Model file for the job. Use its own axes, mm. Coordinates: 2 decimals unless noted, no trailing zeros. Write each loop counter-clockwise with the first axis right and the second up, starting at its lowest first coordinate (ties: lowest second). Pieces come first, ordered by that corner, then holes. Notation, with made-up numbers: (-11.5, 0.5) -> (44.5, 0.5) arc R21 cw to (44.5, 11.5) -> close; hole circle Ø4 at (80.25, -9). An arc over 180 degrees is marked (long way). Answer as a JSON object with one key per item and string values. Group by question number.
from build123d import *

# Parameters (mm, degrees)
SKETCH1_W           = 74.6
SKETCH1_H           = 62
BOSS_EXTRUDE1_DEPTH = 3.2
CUT_EXTRUDE1_REACH  = 5.2
SKETCH2_R           = 21.05
CUT_EXTRUDE2_REACH  = 5.2
SKETCH3_R           = 2.625


with BuildPart() as part:
    # Sketch1 → Boss-Extrude1 (new body)
    with BuildSketch(Plane(origin=(0, 0, 0), x_dir=(0, 0, -1), z_dir=(1, 0, 0))):
        with Locations((37.3, 31)):
            Rectangle(SKETCH1_W, SKETCH1_H)
    extrude(amount=BOSS_EXTRUDE1_DEPTH)

    # Sketch2 → Cut-Extrude1 (cut, up to next)
    with BuildSketch(Plane(origin=(3.2, 0, 0), x_dir=(0, 0, -1), z_dir=(1, 0, 0)), mode=Mode.PRIVATE) as cut_extrude1_sk1:
        with Locations((37.3, 31)):
            Circle(SKETCH2_R)
    cut_extrude1_tool1 = extrude(cut_extrude1_sk1.sketch, amount=-CUT_EXTRUDE1_REACH, mode=Mode.PRIVATE) & part.part
    add(cut_extrude1_tool1.solids().sort_by_distance((3.2, 31, -37.3))[0], mode=Mode.SUBTRACT)

    # Sketch3 → Cut-Extrude2 (cut, up to next)
    with BuildSketch(Plane.ZY, mode=Mode.PRIVATE) as cut_extrude2_sk1:
        with Locations((-67.1, 13)):
            Circle(SKETCH3_R)
    cut_extrude2_tool1 = extrude(cut_extrude2_sk1.sketch, amount=-CUT_EXTRUDE2_REACH, mode=Mode.PRIVATE) & part.part
    add(cut_extrude2_tool1.solids().sort_by_distance((0, 13, -67.1))[0], mode=Mode.SUBTRACT)
    # Sketch3 → Cut-Extrude2 (cut, up to next)
    with BuildSketch(Plane.ZY, mode=Mode.PRIVATE) as cut_extrude2_sk2:
        with Locations((-67.1, 49)):
            Circle(SKETCH3_R)
    cut_extrude2_tool2 = extrude(cut_extrude2_sk2.sketch, amount=-CUT_EXTRUDE2_REACH, mode=Mode.PRIVATE) & part.part
    add(cut_extrude2_tool2.solids().sort_by_distance((0, 49, -67.1))[0], mode=Mode.SUBTRACT)
    # Sketch3 → Cut-Extrude2 (cut, up to next)
    with BuildSketch(Plane.ZY, mode=Mode.PRIVATE) as cut_extrude2_sk3:
        with Locations((-7.5, 13)):
            Circle(SKETCH3_R)
    cut_extrude2_tool3 = extrude(cut_extrude2_sk3.sketch, amount=-CUT_EXTRUDE2_REACH, mode=Mode.PRIVATE) & part.part
    add(cut_extrude2_tool3.solids().sort_by_distance((0, 13, -7.5))[0], mode=Mode.SUBTRACT)
    # Sketch3 → Cut-Extrude2 (cut, up to next)
    with BuildSketch(Plane.ZY, mode=Mode.PRIVATE) as cut_extrude2_sk4:
        with Locations((-7.5, 49)):
            Circle(SKETCH3_R)
    cut_extrude2_tool4 = extrude(cut_extrude2_sk4.sketch, amount=-CUT_EXTRUDE2_REACH, mode=Mode.PRIVATE) & part.part
    add(cut_extrude2_tool4.solids().sort_by_distance((0, 49, -7.5))[0], mode=Mode.SUBTRACT)


solid = part.part
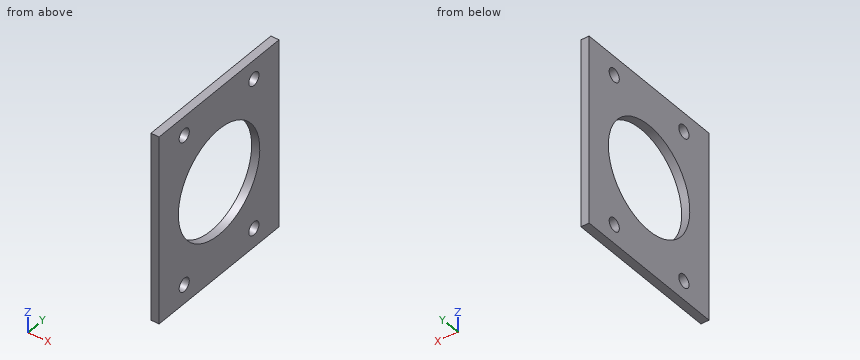
(1) Pin check, flat tip, straight feed: pin 1 (4.5 mm diameter, centred on y = 49, z = -67.1, fed in from +X) (3 decimals). Stop position of the tip, or through.
(2) Cut at A-A on z = -37.3. List the corners of the cut face in (x, y), plus the area to 3 significant figures.
(3) Wall check: probe 1 along Y at (x, z) = (1.7, -67.1) (3 decimals); probe 2 along Z at (x, y) = (1.6, 29); probe 3 along Y at (x, z) = (1.65, -37.3). Give the ranges that are in metal, low to high.
(4) Cut at D-D on y = 31. List the corners of the cut face in (x, z).
(5) Cut at C-C on z = -67.1. List the corners of the cut face in (x, y) (3 decimals), plus the area to 3 significant figures.
(6) Cut at B-B on x = 2.05. List the corners of the cut face in (y, z) (3 decimals), plus the area to 3 significant figures.
Results found:
{
 "1": {"pin 1": "passes through"},
 "2": {"outline": "(0, 0) -> (3.2, 0) -> (3.2, 9.95) -> (0, 9.95) -> close; (0, 52.05) -> (3.2, 52.05) -> (3.2, 62) -> (0, 62) -> close", "area": "63.7 mm²"},
 "3": {"probe 1": "y = 0 to 10.375, 15.625 to 46.375, 51.625 to 62", "probe 2": "z = -74.6 to -58.25, -16.35 to 0", "probe 3": "y = 0 to 9.95, 52.05 to 62"},
 "4": {"outline": "(0, -74.6) -> (3.2, -74.6) -> (3.2, -58.35) -> (0, -58.35) -> close; (0, -16.25) -> (3.2, -16.25) -> (3.2, 0) -> (0, 0) -> close"},
 "5": {"outline": "(0, 0) -> (3.2, 0) -> (3.2, 10.375) -> (0, 10.375) -> close; (0, 15.625) -> (3.2, 15.625) -> (3.2, 46.375) -> (0, 46.375) -> close; (0, 51.625) -> (3.2, 51.625) -> (3.2, 62) -> (0, 62) -> close", "area": "165 mm²"},
 "6": {"outline": "(0, -74.6) -> (62, -74.6) -> (62, 0) -> (0, 0) -> close; hole circle Ø42.1 at (31, -37.3); hole circle Ø5.25 at (13, -67.1); hole circle Ø5.25 at (13, -7.5); hole circle Ø5.25 at (49, -67.1); hole circle Ø5.25 at (49, -7.5)", "area": "3,150 mm²"}
}
